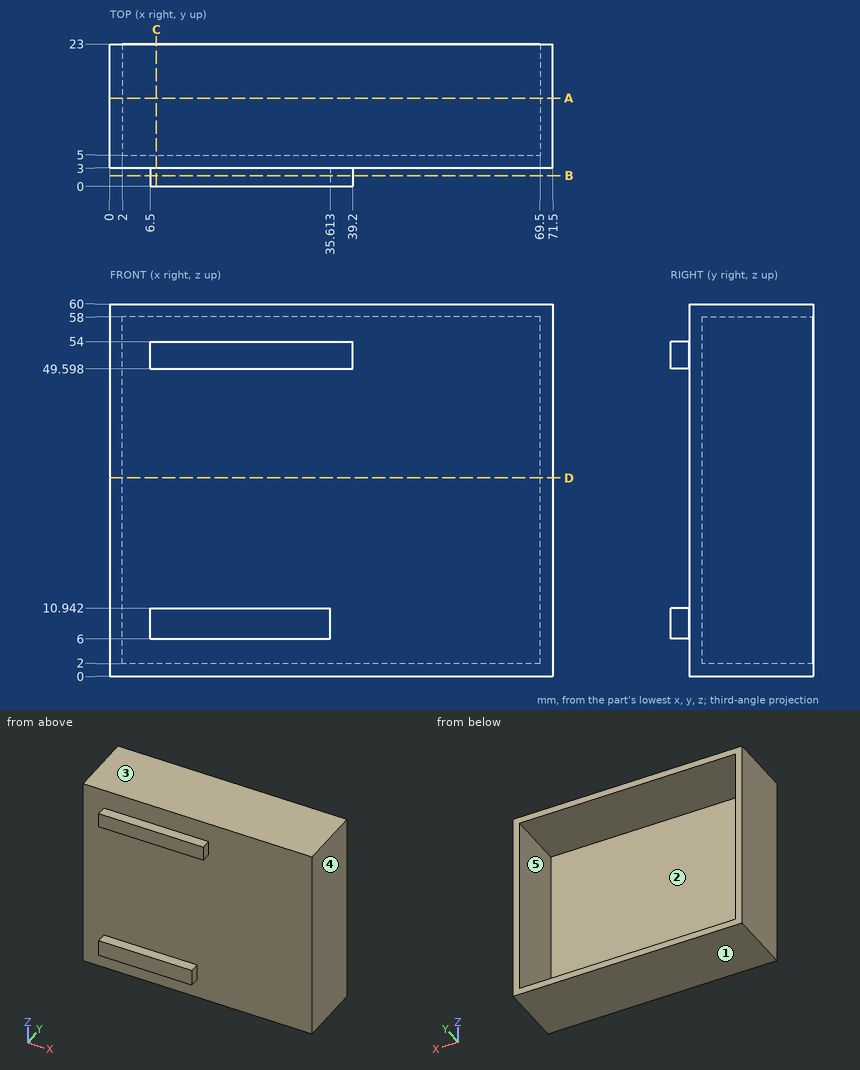
Could you check a few things on this drawing? It's one solid part, dimensions in mm from its lowest x, y, z. A direction names the side the tool comes from. Round coordinates to 2 decimals unless told otherwise and drop trailing zeros. Order: outer loops, then holes, each group sorted by start corner. A loop starts at its lowest first (then second) coordinate and runs counter-clockwise, first axis right, second up. Notation, with made-up numbers: M -15.75,50.5 L 27.25,50.5 A10 cw 27.25,62.5 Z; hole C -24,55.5 d5. An arc over 180 degrees is marked long. One line per item, written item: value.
(1) Imagine slicing it at B-B (y = 1.75). Write out the boundary of the cut face in (x, z), and give its area (3 significant figures).
Ans:
outline: M 6.5,6 L 35.61,6 L 35.61,10.94 L 6.5,10.94 Z; M 6.5,49.6 L 39.2,49.6 L 39.2,54 L 6.5,54 Z
area: 288 mm^2
(2) Imagine slicing it at D-D (z = 32). Write out the boundary of the cut face in (x, y), and give its area (3 significant figures).
Ans:
outline: M 0,3 L 71.5,3 L 71.5,23 L 69.5,23 L 69.5,5 L 2,5 L 2,23 L 0,23 Z
area: 215 mm^2
(3) If we mould it in two halves opening along X, with no side actions, what happens to the marked faces 3, 4 and 5? For each: released by +X, released by -X, zero draft, split by the parting line, or undercut.
Ans:
face 3: zero draft
face 4: released by +X
face 5: undercut
(4) I need wall thicknesses on line 1 along X through (y, z) = (10, 43); line 2 along Z through (x, y) = (34.5, 21.75); line 3 along Y through (x, z) = (46.5, 28). Which ranges of each line are inside material? Lowest first, please. Write a range as from..to.
Ans:
line 1: x = 0..2, 69.5..71.5
line 2: z = 0..2, 58..60
line 3: y = 3..5
(5) Which directions (+Z, -Z, +X, -X, +Y, -Y) give clear straight access to the entire face, cutting with the end or side of a thin tool? Please do the marked faces 1 and 2.
Ans:
face 1: -Z, +X, -X, +Y, -Y
face 2: +Y
(6) Imagine slicing it at A-A (y = 14.25). Write out the boundary of the cut face in (x, z).
Ans:
outline: M 0,0 L 71.5,0 L 71.5,60 L 0,60 Z; hole M 2,2 L 69.5,2 L 69.5,58 L 2,58 Z
(7) Imagine slicing it at C-C (x = 7.5). Write out the boundary of the cut face in (y, z).
Ans:
outline: M 0,6 L 3,6 L 3,0 L 23,0 L 23,2 L 5,2 L 5,58 L 23,58 L 23,60 L 3,60 L 3,54 L 0,54 L 0,49.6 L 3,49.6 L 3,10.94 L 0,10.94 Z
(8) I'm going to push flat-ended pins straight in: P1, Ø6, axis at x = 48.5, z = 36.5, coming from the -Y side; P2, Ø12, axis at x = 31, z = 37, coming from the +Y side; P3, Ø1.5, axis at x = 19.5, y = 1, coming from the +Z side. Where does each tip first touch, or does it pass through?
Ans:
P1: stops at y = 3
P2: stops at y = 5
P3: stops at z = 54
